from build123d import *

# Parameters (mm, degrees)
F0_W      = 86
F0_H      = 14
F1_DEPTH  = 4
F3_DEPTH  = 4
F5_DEPTH  = 2
F6_R      = 0.25
F7_W      = 21.9838
F7_H      = 14
F8_DEPTH  = 4
F9_W      = 4
F9_H      = 14
F10_DEPTH = 18.7753
F11_W     = 14
F11_H     = 4
F12_DEPTH = 40.005
F13_R     = 0.25


with BuildPart() as f1:
    # F0 (on Top) → F1 (new body)
    with BuildSketch(Plane.XY):
        Rectangle(F0_W, F0_H)
    extrude(amount=F1_DEPTH)

    # F2 (on face) → F3 (cut)
    with BuildSketch(Plane.XY.offset(4)):
        with BuildLine():
            ThreePointArc((35, -2), (36.4142139414, -1.4142137697), (37.0000005863, 0))
            ThreePointArc((37.0000005863, 0), (36.4142139414, 1.4142137697), (35, 2))
            Line((35, 2), (35, -2))
        make_face()
        with BuildLine():
            Line((35, -2), (35, 2))
            ThreePointArc((35, 2), (33.0000005863, 0), (35, -2))
        make_face()
        with BuildLine():
            ThreePointArc((35, -2), (33.0000005863, 0), (35, 2))
            Line((35, 2), (11, 2))
            ThreePointArc((11, 2), (12.4142135624, 1.4142135624), (13, 0))
            ThreePointArc((13, 0), (12.4142135624, -1.4142135624), (11, -2))
            Line((11, -2), (35, -2))
        make_face()
        with BuildLine():
            Line((11, -2), (11, 2))
            ThreePointArc((11, 2), (9, 0), (11, -2))
        make_face()
        with BuildLine():
            ThreePointArc((13, 0), (12.4142135624, 1.4142135624), (11, 2))
            Line((11, 2), (11, -2))
            ThreePointArc((11, -2), (12.4142135624, -1.4142135624), (13, 0))
        make_face()
    extrude(amount=-F3_DEPTH, mode=Mode.SUBTRACT)

    # F4 (on face) → F5 (cut)
    with BuildSketch(Plane.XY.offset(4)):
        with BuildLine():
            ThreePointArc((35.0000005863, -4), (37.8284277111, -2.8284271247), (39.0000005863, 0))
            ThreePointArc((39.0000005863, 0), (37.8284277111, 2.8284271247), (35.0000005863, 4))
            Line((35.0000005863, 4), (35.0000005863, -4))
        make_face()
        with BuildLine():
            Line((35.0000005863, -4), (35.0000005863, 4))
            ThreePointArc((35.0000005863, 4), (31.0000005863, 0), (35.0000005863, -4))
        make_face()
        with BuildLine():
            ThreePointArc((35.0000005863, -4), (31.0000005863, 0), (35.0000005863, 4))
            Line((35.0000005863, 4), (11.0000005863, 4))
            ThreePointArc((11.0000005863, 4), (13.828427332, 2.8284269175), (15, 0))
            ThreePointArc((15, 0), (13.828427332, -2.8284269175), (11.0000005863, -4))
            Line((11.0000005863, -4), (35.0000005863, -4))
        make_face()
        with BuildLine():
            Line((11.0000005863, -4), (11.0000005863, 4))
            ThreePointArc((11.0000005863, 4), (7, 0), (11.0000005863, -4))
        make_face()
        with BuildLine():
            ThreePointArc((15, 0), (13.828427332, 2.8284269175), (11.0000005863, 4))
            Line((11.0000005863, 4), (11.0000005863, -4))
            ThreePointArc((11.0000005863, -4), (13.828427332, -2.8284269175), (15, 0))
        make_face()
    extrude(amount=-F5_DEPTH, mode=Mode.SUBTRACT)

    # F6
    f6_edges = [f1.edges().sort_by_distance(p)[0] for p in [
        (23.000001, 4, 2),
        (7, 0, 2),
        (23.000001, -4, 2),
        (39.000001, 0, 2),
        (23.000001, -4, 4),
        (7, 0, 4),
        (23.000001, 4, 4),
        (39.000001, 0, 4),
    ]]
    fillet(f6_edges, radius=F6_R)

    # F7 (on face) → F8 (cut)
    with BuildSketch(Plane.XY.offset(4)):
        with Locations((-32.0081, 0)):
            Rectangle(F7_W, F7_H)
    extrude(amount=-F8_DEPTH, mode=Mode.SUBTRACT)

    # F9 (on face) → F10 (join)
    with BuildSketch(Plane(origin=(0, 0, 0), x_dir=(1, 0, 0), z_dir=(0, 0, -1))):
        with Locations((-19.0162, 0)):
            Rectangle(F9_W, F9_H)
    extrude(amount=F10_DEPTH)

    # F11 (on face) → F12 (join)
    with BuildSketch(Plane(origin=(-21.0162, 0, 0), x_dir=(0, -1, 0), z_dir=(-1, 0, 0))):
        with Locations((0, -16.7753)):
            Rectangle(F11_W, F11_H)
    extrude(amount=F12_DEPTH)

    # F13
    f13_edges = [f1.edges().sort_by_distance(p)[0] for p in [
        (-17.0162, 0, 0),
        (-17.0162, 0, -18.7753),
        (43, 0, 0),
        (43, 0, 4),
        (-21.0162, 0, -14.7753),
        (-21.0162, 0, 4),
        (-61.0212, 0, -14.7753),
        (-61.0212, 0, -18.7753),
    ]]
    fillet(f13_edges, radius=F13_R)


solid = f1.part
Build history of the part. All positions in model axes, mm. A direction names the side the tool comes from. Round coordinates to 2 decimals unless told otherwise and drop trailing zeros. Write each loop counter-clockwise with the first axis right and the second up, starting at its lowest first coordinate (ties: lowest second). Pieces come first, ordered by that corner, then holes. Notation, with made-up numbers: (-38.75, 75) - (-14.75, 75) arc R24 ccw to (-14.75, 96) - close; hole circle Ø5 at (64, -17). An arc over 180 degrees is marked (long way). One line per question, with ' | ' between items.
1. Band-saw the part on B-B, the plane y = 5.75. Write the cut outline in (x, z).
Results are:
outline: (-61.02, -18.53) arc R0.25 ccw to (-60.77, -18.78) - (-17.27, -18.78) arc R0.25 ccw to (-17.02, -18.53) - (-17.02, -0.25) arc R0.25 cw to (-16.77, 0) - (42.75, 0) arc R0.25 ccw to (43, 0.25) - (43, 3.75) arc R0.25 ccw to (42.75, 4) - (-20.77, 4) arc R0.25 ccw to (-21.02, 3.75) - (-21.02, -14.53) arc R0.25 cw to (-21.27, -14.78) - (-60.77, -14.78) arc R0.25 ccw to (-61.02, -15.03) - close
2. Band-saw the part on D-D, the plane z = -4.5. Write the cut outline in (x, y), and give its area (3 significant figures).
Results are:
outline: (-21.02, -7) - (-17.02, -7) - (-17.02, 7) - (-21.02, 7) - close | area: 56.0 mm^2
3. Mould opens along Y. For faces 6 (the face through (13, 3, 0)), 7 (the face through (7, 0, 3)), 8 (the face through (-8.8, 7, 0.2)) say: released by +Y, released by -Y, zero draft, split by the parting line, or undercut.
Results are:
face 6: zero draft | face 7: undercut | face 8: released by +Y
4. Drop flat-ended pins along their axis: pin 1 Ø4 at (x, y) = (10.5, -2) entering from -Z; pin 2 Ø3 at (x, y) = (-44, 2.5) entering from +Z; pin 3 Ø7 at (y, z) = (2.5, -8.5) entering from +X. Give the stop position or say it passes through.
Results are:
pin 1: z = 0 | pin 2: z = -14.78 | pin 3: x = -17.02
5. Tool access for faces 1 (the face through (3, 0, 4)), 2 (the face through (-21.016, 0, -5)), 3 (the face through (23, -2, 1)), 4 (the face through (22.8, -2.4, 2)), 5 (the face through (-17.016, 0, -9)): list every direction of +Z, -Z, +X, -X, +Y, -Y with a clear straight run to the whole face (end or side of a thin tool).
Results are:
face 1: +Z, +X, -X, +Y, -Y | face 2: +Z, -X, +Y, -Y | face 3: +Z, -Z | face 4: +Z | face 5: -Z, +X, +Y, -Y
6. Band-saw the part on C-C, the plane z = -16. Write the cut outline in (x, y).
Results are:
outline: (-61.02, -7) - (-17.02, -7) - (-17.02, 7) - (-61.02, 7) - close
7. Band-saw the part on A-A, the plane x = 12.5. Write the cut outline in (y, z), and give its area (3 significant figures).
Results are:
outline: (-7, 0) - (-2, 0) - (-2, 2) - (-3.75, 2) arc R0.25 cw to (-4, 2.25) - (-4, 3.75) arc R0.25 ccw to (-4.25, 4) - (-7, 4) - close; (2, 0) - (7, 0) - (7, 4) - (4.25, 4) arc R0.25 ccw to (4, 3.75) - (4, 2.25) arc R0.25 cw to (3.75, 2) - (2, 2) - close | area: 32.0 mm^2
8. Drill centre lines: line 1 along X through (y, z) = (-6, -3.75); line 2 along Z through (x, y) = (-15, -2.75); line 3 along Z through (x, y) = (-46, -2). Where is each one in solid material? Low to high. Write a range as from..to.
Results are:
line 1: -21.02..-17.02 | line 2: 0..4 | line 3: -18.78..-14.78
